Autodesk Inventor part; units mm, degrees
ref_plane "YZ Plane" through (0, 0, 0) normal (1, 0, 0) x (0, 1, 0)
ref_plane "XZ Plane" through (0, 0, 0) normal (0, 1, 0) x (-1, 0, 0)
ref_plane "XY Plane" through (0, 0, 0) normal (0, 0, 1) x (1, 0, 0)
sketch "Sketch1" plane through (0, 0, 0) normal (0, 0, 1) x (1, 0, 0)
  line L0 (0, 0) -> (70, 0)
  line L1 (70, 0) -> (70, -120)
  line L2 (70, -120) -> (0, -120)
  line L3 (0, -120) -> (0, 0)
  dimension "d0" = 70
  dimension "d1" = 120
extrude "Extrusion1" add sketch "Sketch1" along normal blind 7.4
sketch "Sketch2" plane through (0, 0, 7.4) normal (0, 0, 1) x (1, 0, 0)
  circle A0 centre (10, -104) radius 2.6
  circle A1 centre (16, -110) radius 2.6
  circle A2 centre (35, -110) radius 2.6
  circle A3 centre (10, -66) radius 2.6
  circle A4 centre (16, -60) radius 2.6
  circle A5 centre (10, -35) radius 2.6
  circle A6 centre (10, -16) radius 2.6
  circle A7 centre (16, -10) radius 2.6
  circle A8 centre (35, -60) radius 2.6
  circle A9 centre (60, -104) radius 2.6
  circle A10 centre (60, -66) radius 2.6
  circle A11 centre (10, -85) radius 2.6
  circle A12 centre (60, -85) radius 2.6
  circle A13 centre (54, -110) radius 2.6
  circle A14 centre (54, -60) radius 2.6
  circle A15 centre (60, -54) radius 2.6
  circle A16 centre (60, -16) radius 2.6
  circle A17 centre (10, -54) radius 2.6
  circle A18 centre (35, -10) radius 2.6
  circle A19 centre (54, -10) radius 2.6
  line L0 (0, 0) -> (0, -120)
  line L1 (70, -120) -> (70, 0)
  line L2 (70, 0) -> (0, 0)
  line L3 (0, -120) -> (70, -120)
  circle A20 centre (60, -35) radius 2.6
  dimension "d5" = 5.2
  dimension "d6" = 5.2
  dimension "d7" = 5.2
  dimension "d10" = 5.2
  dimension "d11" = 5.2
  dimension "d12" = 5.2
  dimension "d15" = 5.2
  dimension "d16" = 5.2
  dimension "d17" = 5.2
  dimension "d19" = 5.2
  dimension "d20" = 5.2
  dimension "d21" = 5.2
  dimension "d22" = 5.2
  dimension "d23" = 5.2
  dimension "d24" = 5.2
  dimension "d25" = 5.2
  dimension "d26" = 5.2
  dimension "d27" = 5.2
  dimension "d54" = 10
  dimension "d55" = 10
  dimension "d56" = 16
  dimension "d57" = 16
  dimension "d58" = 16
  dimension "d59" = 35
  dimension "d60" = 10
  dimension "d61" = 19
  dimension "d62" = 19
  dimension "d63" = 19
  dimension "d64" = 5.2
  dimension "d67" = 6
  dimension "d68" = 6
  dimension "d69" = 6
  dimension "d70" = 6
  dimension "d71" = 19
  dimension "d72" = 19
  dimension "d74" = 6
  dimension "d75" = 10
extrude "Extrusion2" cut sketch "Sketch2" against normal through all contours A0 | A1 | A2 | A3 | A4 | A5 | A6 | A7 | A8 | A9 | A10 | A11 | A12 | A13 | A14 | A15 | A16 | A17 | A18 | A19 | A20
sketch "Sketch3" plane through (0, 0, 7.4) normal (0, 0, 1) x (1, 0, 0)
  line L0 (15, -15) -> (55, -15)
  line L1 (55, -15) -> (55, -55)
  line L2 (55, -55) -> (15, -55)
  line L3 (15, -55) -> (15, -15)
  line L4 (15, -65) -> (55, -65)
  line L5 (55, -65) -> (55, -105)
  line L6 (55, -105) -> (15, -105)
  line L7 (15, -105) -> (15, -65)
  line L8 (0, 0) -> (0, -120)
  line L9 (70, 0) -> (0, 0)
  line L10 (0, -120) -> (70, -120)
  line L11 (70, -120) -> (70, 0)
  circle A0 centre (35, -10) radius 2.6
  circle A1 centre (35, -60) radius 2.6
  line L12 (5, -5) -> (65, -5)
  line L13 (65, -5) -> (65, -115)
  line L14 (65, -115) -> (5, -115)
  line L15 (5, -115) -> (5, -5)
  circle A2 centre (16, -10) radius 2.6
  circle A3 centre (60, -16) radius 2.6
  circle A4 centre (10, -35) radius 2.6
  circle A5 centre (35, -110) radius 2.6
  dimension "d47" = 15
  dimension "d48" = 15
  dimension "d76" = 15
  dimension "d77" = 15
  dimension "d78" = 15
  dimension "d80" = 5
  dimension "d81" = 5
  dimension "d82" = 5
  dimension "d83" = 5
  dimension "d84" = 5
  dimension "d85" = 5
extrude "Extrusion3" cut sketch "Sketch3" against normal blind 5.9 contours L0 L1 L2 L3 | L4 L5 L6 L7 | L9 L11 L10 L8
fillet "Fillet1" radius 10 2 edges at (70, 0, 0.75) (0, 0, 0.75)
fillet "Fillet2" radius 10 2 edges at (65, -5, 4.45) (5, -5, 4.45)
properties part number "edition 2"
Source: CAD feature listing. Evaluate the final solid. Frame: model axes, mm. A direction names the side the tool comes from. Give positions to 0.01 mm unless a question says otherwise; leave off trailing zeros. Write each loop counter-clockwise with the first axis right and the second up, starting at its lowest first coordinate (ties: lowest second). Pieces come first, ordered by that corner, then holes.
1. Material intervals for line 1 along Y through (x, z) = (35, 3.25); line 2 along X through (y, z) = (-93.5, 4); line 3 along Y through (x, z) = (17.5, 4.75), sorted ascending.
2. Access query for faces 4 (the face through (15, -85, 4)), 5 (the face through (9.662, -82.422, 3.752)), 6 (the face through (61.99, -7.85, 4.41)). Directions: +Z, -Z, +X, -X, +Y, -Y. A direction counts if a zero-diameter tool reaches every point of the face in a straight line with its end or side. Return the directions, or none.
3. First-contact query: pin 1 (2 mm diameter, centred on x = 20.5, y = -85.5, fed in from +Z); pin 2 (1.8 mm diameter, centred on x = 32.5, z = 3.5, fed in from +Y); pin 3 (3 mm diameter, centred on x = 29.5, z = 5, fed in from -Y). Flat tips, straight axial feed; report the tip coordinate or a pass-through.
4. Section query D-D (z = 3.5). Count the separate pieces of the cut face and the enclosed holes in it, then the cut area to 3 significant figures.
5. Section query C-C (y = -23.5). Return the cut outline in (x, z).
6. Pull-direction query (X, two-part tool) for faces 1 (the face through (33.084, -58.243, 3.752)), 2 (the face through (3.01, -2.85, 0.76)), 3 (the face through (65, -64, 4)); classes: +X half, -X half, draft (parallel to the pull), parting line (faces both ways), or undercut.
7. Section query B-B (x = 35). Return the cut outline in (y, z).
8. Section query A-A (y = -60). Return the cut outline in (x, z).
Output values:
1. line 1: y = -115 to -112.6, -107.4 to -105, -65 to -62.6, -57.4 to -55, -15 to -12.6, -7.4 to -5
1. line 2: x = 5 to 15, 55 to 65
1. line 3: y = -115 to -112.12, -107.88 to -105, -65 to -62.12, -57.88 to -55, -15 to -12.12, -7.88 to -5
2. face 4: +Z
2. face 5: +Z, -Z
2. face 6: +Z, +X, +Y
3. pin 1: stops at z = 1.5
3. pin 2: stops at y = -5
3. pin 3: stops at y = -115
4. separate pieces: 1
4. enclosed holes: 23
4. area: 2,910 mm2
5. outline: (0, 0) - (70, 0) - (70, 1.5) - (65, 1.5) - (65, 7.4) - (55, 7.4) - (55, 1.5) - (15, 1.5) - (15, 7.4) - (5, 7.4) - (5, 1.5) - (0, 1.5) - close
6. face 1: undercut
6. face 2: -X half
6. face 3: +X half
7. outline: (-120, 0) - (-112.6, 0) - (-112.6, 7.4) - (-115, 7.4) - (-115, 1.5) - (-120, 1.5) - close; (-107.4, 0) - (-62.6, 0) - (-62.6, 7.4) - (-65, 7.4) - (-65, 1.5) - (-105, 1.5) - (-105, 7.4) - (-107.4, 7.4) - close; (-57.4, 0) - (-12.6, 0) - (-12.6, 7.4) - (-15, 7.4) - (-15, 1.5) - (-55, 1.5) - (-55, 7.4) - (-57.4, 7.4) - close; (-7.4, 0) - (0, 0) - (0, 1.5) - (-5, 1.5) - (-5, 7.4) - (-7.4, 7.4) - close
8. outline: (0, 0) - (13.4, 0) - (13.4, 7.4) - (5, 7.4) - (5, 1.5) - (0, 1.5) - close; (18.6, 0) - (32.4, 0) - (32.4, 7.4) - (18.6, 7.4) - close; (37.6, 0) - (51.4, 0) - (51.4, 7.4) - (37.6, 7.4) - close; (56.6, 0) - (70, 0) - (70, 1.5) - (65, 1.5) - (65, 7.4) - (56.6, 7.4) - close
